Geometry check sheet. Reference: the model listing, model coordinates, mm. A direction names the side the tool comes from. Round coordinates to 2 decimals unless told otherwise and drop trailing zeros. Write each loop counter-clockwise with the first axis right and the second up, starting at its lowest first coordinate (ties: lowest second). Pieces come first, ordered by that corner, then holes. Notation, with made-up numbers: M 82,-35 L 104,-35 A20 ccw 104,-23 Z; hole C 39,-24.75 d3. An arc over 180 degrees is marked long. Put each result on its own line as item: value. Start each with the question number.
(1) Section check D-D on z = 5. Count the separate pieces of the cut face and the enclosed holes in it, then the cut area to 3 significant figures.
(2) Section check A-A on x = 0. Record the cut outline in (y, z) (3 decimals), then the cut area to 3 significant figures.
(3) Section check B-B on y = 0. Record the cut outline in (x, z).
(4) Mould release check, pull along X, two halves, no side actions. Record for faces 1 (the flat face through (-28, -6.585, 4)), 2 (the cylindrical face through (-39.021, -22.414, 3.451)): pulls with the +X half, pulls with the -X half, needs draft (parallel to the pull), parting line crosses it, or undercut.
(5) Gauge pin test, flat ends, axial feed: pin 1 (2 mm diameter, centred on x = -6.5, y = 24, fed in from -Z); pin 2 (1.5 mm diameter, centred on x = 3.5, z = 2.5, fed in from -Y); pin 3 (2 mm diameter, centred on y = 26, z = 1.5, fed in from +X); pin 4 (3 mm diameter, centred on y = 26, z = 4, fed in from -X). Record the tip position at first contact, or that the pin passes through.
(6) Section check C-C on x = 19. Record the cut outline in (y, z), then the cut area to 3 significant figures.
(7) Tool access check on faces 3 (the flat face through (0, 41.415, 4)), 4 (the cylindrical face through (-12.709, 18.225, 3.451)). Record the directions out of +Z, -Z, +X, -X, +Y, -Y that give a thin tool (end or side, any length) a straight path to the whole face; none if there is none.
(8) Material ranges on probe 1 along Y at (x, z) = (0, 4) (3 decimals); probe 2 along Y at (x, z) = (2.5, 3.25) (3 decimals); probe 3 along Y at (x, z) = (27, 1.5) (3 decimals), recorded low to high.
from build123d import *

# Parameters (mm, degrees)
F0_R     = 11
F1_DEPTH = 7
F3_DEPTH = 25


with BuildPart() as f1:
    # F0 (on Top) → F1 (new body)
    with BuildSketch(Plane.XY):
        with BuildLine():
            ThreePointArc((-16.867813, -23.168401), (-9.341205, -20.041676), (-5.337589, -12.942571))
            ThreePointArc((-5.337589, -12.942571), (-12.124356, -7), (-13.87739, 1.848798))
            ThreePointArc((-13.87739, 1.848798), (-22.027203, 1.931118), (-28.49833, -3.023754))
            ThreePointArc((-28.49833, -3.023754), (-29.433898, -3.114432), (-30.360469, -3.272474))
            ThreePointArc((-30.360469, -3.272474), (-33.819311, -2.907046), (-35.762261, -5.791847))
            ThreePointArc((-35.762261, -5.791847), (-39.059816, -6.445953), (-39.142749, -9.806733))
            ThreePointArc((-39.142749, -9.806733), (-41.985912, -12.202508), (-40.709221, -15.694408))
            ThreePointArc((-40.709221, -15.694408), (-38.971143, -22.5), (-33.946366, -27.408015))
            ThreePointArc((-33.946366, -27.408015), (-31.560638, -30.259612), (-28.064255, -28.995249))
            ThreePointArc((-28.064255, -28.995249), (-25.112267, -30.603816), (-22.897017, -28.075103))
            ThreePointArc((-22.897017, -28.075103), (-19.427231, -27.83486), (-18.01428, -24.6567))
            ThreePointArc((-18.01428, -24.6567), (-17.414126, -23.933288), (-16.867813, -23.168401))
        make_face()
        with BuildLine():
            ThreePointArc((5.337589, -12.942571), (11.634566, -7.786968), (14, 0))
            ThreePointArc((14, 0), (13.969314, 0.92643), (13.87739, 1.848798))
            ThreePointArc((13.87739, 1.848798), (12.124356, 7), (8.539801, 11.093773))
            ThreePointArc((8.539801, 11.093773), (0, 14), (-8.539801, 11.093773))
            ThreePointArc((-8.539801, 11.093773), (-12.124356, 7), (-13.87739, 1.848798))
            ThreePointArc((-13.87739, 1.848798), (-12.124356, -7), (-5.337589, -12.942571))
            ThreePointArc((-5.337589, -12.942571), (0, -14), (5.337589, -12.942571))
        make_face()
        Circle(F0_R, mode=Mode.SUBTRACT)
        with BuildLine():
            ThreePointArc((13.87739, 1.848798), (13.969314, 0.92643), (14, 0))
            ThreePointArc((14, 0), (11.634566, -7.786968), (5.337589, -12.942571))
            ThreePointArc((5.337589, -12.942571), (9.341205, -20.041676), (16.867813, -23.168401))
            ThreePointArc((16.867813, -23.168401), (17.414126, -23.933288), (18.01428, -24.6567))
            ThreePointArc((18.01428, -24.6567), (19.427231, -27.83486), (22.897017, -28.075103))
            ThreePointArc((22.897017, -28.075103), (25.112267, -30.603816), (28.064255, -28.995249))
            ThreePointArc((28.064255, -28.995249), (31.560638, -30.259612), (33.946366, -27.408015))
            ThreePointArc((33.946366, -27.408015), (38.971143, -22.5), (40.709221, -15.694408))
            ThreePointArc((40.709221, -15.694408), (41.985912, -12.202508), (39.142749, -9.806733))
            ThreePointArc((39.142749, -9.806733), (39.059816, -6.445953), (35.762261, -5.791847))
            ThreePointArc((35.762261, -5.791847), (33.819311, -2.907046), (30.360469, -3.272474))
            ThreePointArc((30.360469, -3.272474), (29.433898, -3.114432), (28.49833, -3.023754))
            ThreePointArc((28.49833, -3.023754), (22.027203, 1.931118), (13.87739, 1.848798))
        make_face()
        with BuildLine():
            ThreePointArc((-8.539801, 11.093773), (0, 14), (8.539801, 11.093773))
            ThreePointArc((8.539801, 11.093773), (12.685998, 18.110559), (11.630517, 26.192155))
            ThreePointArc((11.630517, 26.192155), (12.019772, 27.04772), (12.346189, 27.929174))
            ThreePointArc((12.346189, 27.929174), (14.39208, 30.741906), (12.865244, 33.86695))
            ThreePointArc((12.865244, 33.86695), (13.947549, 37.049769), (11.078495, 38.801982))
            ThreePointArc((11.078495, 38.801982), (10.425274, 42.46212), (6.762854, 43.102423))
            ThreePointArc((6.762854, 43.102423), (0, 45), (-6.762854, 43.102423))
            ThreePointArc((-6.762854, 43.102423), (-10.425274, 42.46212), (-11.078495, 38.801982))
            ThreePointArc((-11.078495, 38.801982), (-13.947549, 37.049769), (-12.865244, 33.86695))
            ThreePointArc((-12.865244, 33.86695), (-14.39208, 30.741906), (-12.346189, 27.929174))
            ThreePointArc((-12.346189, 27.929174), (-12.019772, 27.04772), (-11.630517, 26.192155))
            ThreePointArc((-11.630517, 26.192155), (-12.685998, 18.110559), (-8.539801, 11.093773))
        make_face()
    extrude(amount=F1_DEPTH)

    # F2 (on face) → F3 (cut)
    with BuildSketch(Plane.XY.offset(7)):
        Polygon((5.435753, 41.415), (-5.435753, 41.415), (-10.871506, 32), (-5.435753, 22.585), (5.435753, 22.585), (10.871506, 32), align=None)
        Polygon((-38.584318, -16), (-33.148566, -25.415), (-22.27706, -25.415), (-16.841307, -16), (-22.27706, -6.585), (-33.148566, -6.585), align=None)
        Polygon((33.148566, -25.415), (38.584318, -16), (33.148566, -6.585), (22.27706, -6.585), (16.841307, -16), (22.27706, -25.415), align=None)
    extrude(amount=-F3_DEPTH, mode=Mode.SUBTRACT)


solid = f1.part
Answers follow:
1. separate pieces: 1
1. enclosed holes: 4
1. area: 1,660 mm^2
2. outline: M -14,0 L -11,0 L -11,7 L -14,7 Z; M 11,0 L 22.585,0 L 22.585,7 L 11,7 Z; M 41.415,0 L 45,0 L 45,7 L 41.415,7 Z
2. area: 127 mm^2
3. outline: M -25.67,0 L -11,0 L -11,7 L -25.67,7 Z; M 11,0 L 25.67,0 L 25.67,7 L 11,7 Z
4. face 1: undercut
4. face 2: pulls with the -X half
5. pin 1: stops at z = 0
5. pin 2: stops at y = -13.73
5. pin 3: stops at x = 12.15
5. pin 4: stops at x = -12.32
6. outline: M -27.48,0 L -19.74,0 L -19.74,7 L -27.48,7 Z; M -12.26,0 L 2.54,0 L 2.54,7 L -12.26,7 Z
6. area: 158 mm^2
7. face 3: +Z, -Z
7. face 4: +Z, -Z, -X
8. probe 1: y = -14 to -11, 11 to 22.585, 41.415 to 45
8. probe 2: y = -13.775 to -10.712, 10.712 to 22.585, 41.415 to 44.757
8. probe 3: y = -30.242 to -25.415, -6.585 to -1.174
